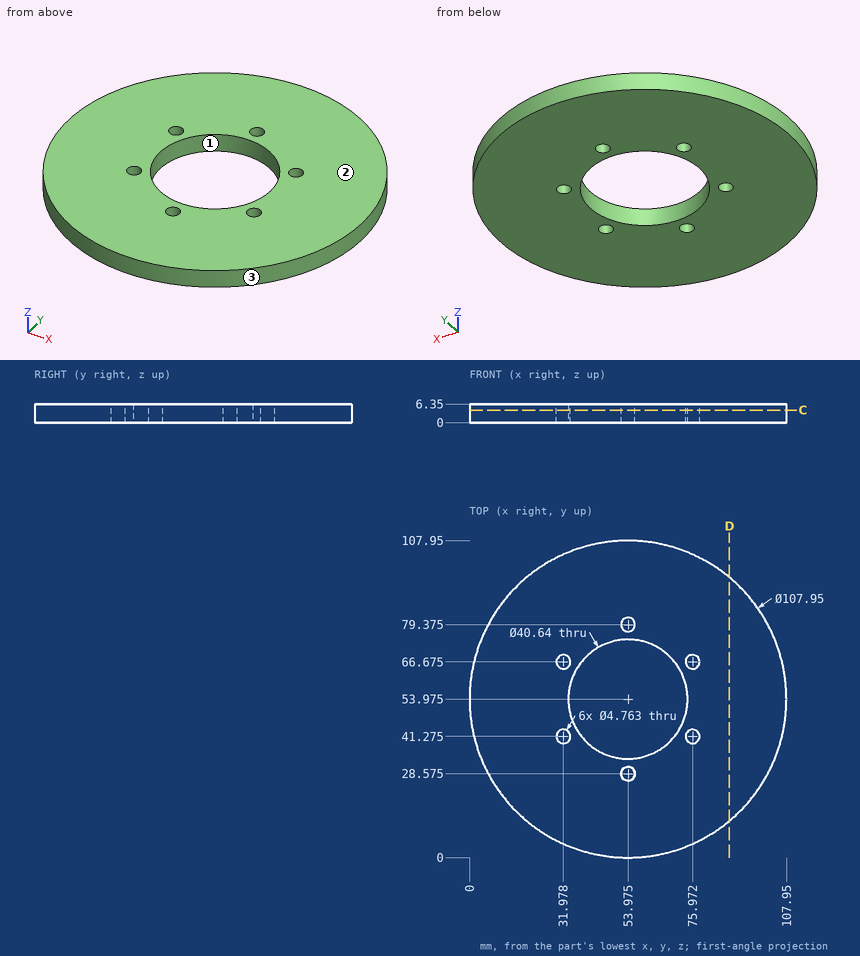
Check sheet for the drawn part. Datum: minimum x, y, z corner. Units: mm. Give positions to 0.01 mm unless a question says otherwise; leave off trailing zeros. Order: outer loops, then holes, each group sorted by start corner. A loop starts at its lowest first (then second) coordinate and runs counter-clockwise, first axis right, second up. Notation, with made-up numbers: (24.5, 48.25) -> (73.5, 48.25) arc R15 cw to (73.5, 54.25) -> close; hole circle Ø9 at (-19.5, 73). An arc over 180 degrees is marked (long way). Answer as CSV lines item,"result".
Q1. Sectioned sample at D-D on x = 88.5. Record the cut outline in (y, z), plus the area to 3 significant figures.
Solutions:
outline,"(12.49, 0) -> (95.46, 0) -> (95.46, 6.35) -> (12.49, 6.35) -> close"
area,"527 mm²"
Q2. Depth check by flat-ended pin: pin 1 (2 mm diameter, centred on y = 69.5, z = 5, fed in from +X); pin 2 (4.5 mm diameter, centred on x = 53.975, y = 79.375, fed in from +Z); pin 3 (1.5 mm diameter, centred on y = 70, z = 2, fed in from -X). Enter the tip coordinate at first touch or a pass-through.
Solutions:
pin 1,"stops at x = 105.96"
pin 2,"passes through"
pin 3,"stops at x = 2.21"
Q3. Scan lines: probe 1 along X at (y, z) = (67, 2.5) (1 decimal); probe 2 along X at (y, z) = (53.5, 4.5); probe 3 along X at (y, z) = (42.5, 2.5) (1 decimal). Record each from-to range of solid material in increasing order.
Solutions:
probe 1,"x = 1.6 to 29.6, 34.3 to 38.4, 69.6 to 73.6, 78.3 to 106.4"
probe 2,"x = 0 to 33.66, 74.29 to 107.95"
probe 3,"x = 1.2 to 29.9, 34 to 37.2, 70.7 to 73.9, 78 to 106.7"
Q4. Release check for a two-part mould opening along Y. For the marked faces 1, 2 and 3 record: +Y half, -Y half, draft (parallel to the pull), parting line (faces both ways), or undercut.
Solutions:
face 1,"undercut"
face 2,"draft"
face 3,"parting line"
Q5. Sectioned sample at C-C on z = 4.25. Count the separate pieces of the cut face and the enclosed holes in it, plus the area to 3 significant figures.
Solutions:
separate pieces,"1"
enclosed holes,"7"
area,"7,750 mm²"
